Can you work these out from the drawing? Everything is in mm from the part's minimum corner. Coordinates: 2 decimals unless noted, no trailing zeros. Loops run counter-clockwise (first coordinate to the right, second up) from the corner with the lowest first, then second, coordinate; pieces in that order, holes last. Notation, with made-up numbers: (-26, -11.5) -> (12, -11.5) arc R29 cw to (12, 16.5) -> close; hole circle Ø10 at (-39.75, 26.25). An arc over 180 degrees is marked (long way). Put each result on its own line as item: value. Start each with the question number.
Item 1: If we section it at C-C on x = 5.25: Please give me the cut outline in (y, z).
Item 2: If we section it at A-A on z = 1.55: Please give me the cut outline in (x, y).
Item 3: Will these pins go through, and if not, where does the flat tip stop? P1, Ø5, axis at x = 28.5, y = 34, coming from the -Z side; P2, Ø0.8, axis at y = 16, z = 1, coming from the +X side.
Item 4: If we section it at D-D on y = 34.5: Please give me the cut outline in (x, z), plus the area to 3 significant figures.
Item 5: Please list where these lines run through material, in increasing order: L1, parallel to X at y = 65.5, z = 1.85; L2, parallel to X at y = 37, z = 1.95; L3, parallel to Y at x = 5, z = 1.8. Write a range as from..to.
Item 6: If we section it at B-B on y = 65.5: Please give me the cut outline in (x, z), plus the area to 3 significant figures.
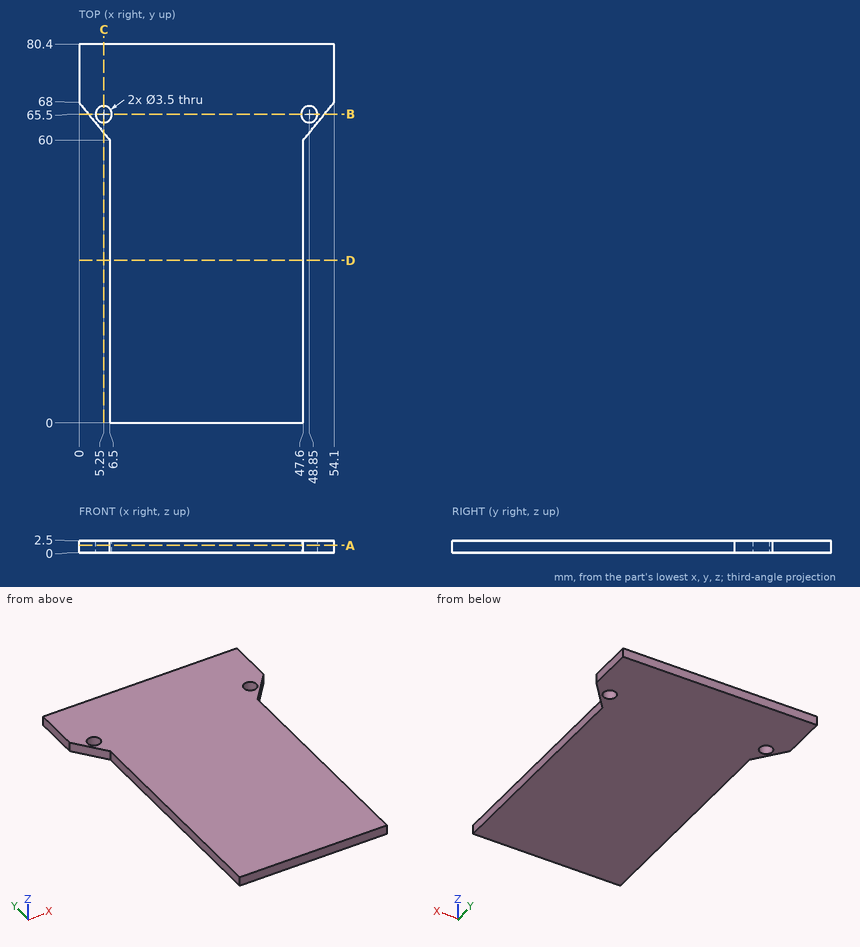
Solutions:
1. outline: (61.54, 0) -> (63.75, 0) -> (63.75, 2.5) -> (61.54, 2.5) -> close; (67.25, 0) -> (80.4, 0) -> (80.4, 2.5) -> (67.25, 2.5) -> close
2. outline: (0, 68) -> (6.5, 60) -> (6.5, 0) -> (47.6, 0) -> (47.6, 60) -> (54.1, 68) -> (54.1, 80.4) -> (0, 80.4) -> close; hole circle Ø3.5 at (5.25, 65.5); hole circle Ø3.5 at (48.85, 65.5)
3. P1: z = 0
3. P2: x = 47.6
4. outline: (6.5, 0) -> (47.6, 0) -> (47.6, 2.5) -> (6.5, 2.5) -> close
4. area: 103 mm^2
5. L1: 2.03..3.5, 7..47.1, 50.6..52.07
5. L2: 6.5..47.6
5. L3: 61.85..63.77, 67.23..80.4
6. outline: (2.03, 0) -> (3.5, 0) -> (3.5, 2.5) -> (2.03, 2.5) -> close; (7, 0) -> (47.1, 0) -> (47.1, 2.5) -> (7, 2.5) -> close; (50.6, 0) -> (52.07, 0) -> (52.07, 2.5) -> (50.6, 2.5) -> close
6. area: 108 mm^2
